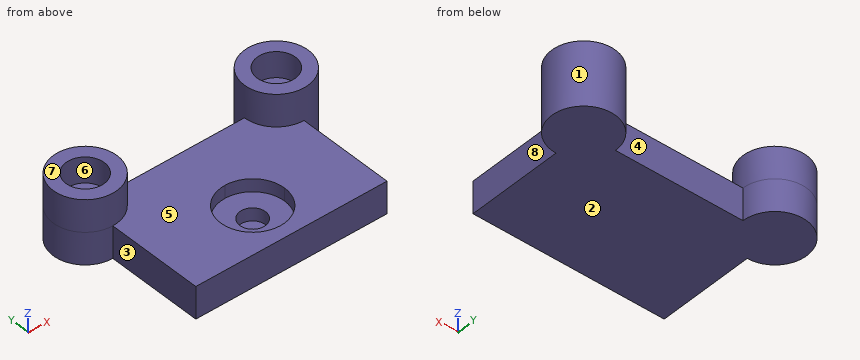
```python
from build123d import *

# Parameters (mm, degrees)
SKETCH_1_W          = 150
SKETCH_1_H          = 100
EXTRUDE_1_DEPTH     = 25
SKETCH_2_R          = 25
EXTRUDE_2_DEPTH     = 25
SKETCH_3_R          = 15
CUT_EXTRUDE_1_DEPTH = 20
SKETCH_4_R          = 7.5
CUT_EXTRUDE_2_DEPTH = 15
CUT_EXTRUDE_3_DEPTH = 10
SKETCH_6_R          = 10
CUT_EXTRUDE_4_DEPTH = 10


with BuildPart() as part:
    # Эскиз1 → Бобышка-Вытянуть1 (new body)
    with BuildSketch(Plane.XY):
        with Locations((75, -50)):
            Rectangle(SKETCH_1_W, SKETCH_1_H)
    extrude(amount=EXTRUDE_1_DEPTH)

    # Эскиз2 → Бобышка-Вытянуть2 (add, symmetric)
    with BuildSketch(Plane.XY.offset(25)):
        Circle(SKETCH_2_R)
        with Locations(Location((150, 0, 0), (0, 0, 180))):
            Circle(SKETCH_2_R)
    extrude(amount=EXTRUDE_2_DEPTH, both=True)

    # Эскиз3 → Вырез-Вытянуть1 (cut)
    with BuildSketch(Plane.XY.offset(50)):
        Circle(SKETCH_3_R)
        with Locations(Location((150, 0, 0), (0, 0, 180))):
            Circle(SKETCH_3_R)
    extrude(amount=-CUT_EXTRUDE_1_DEPTH, mode=Mode.SUBTRACT)

    # Эскиз4 → Вырез-Вытянуть2 (cut)
    with BuildSketch(Plane.XY.offset(30)):
        Circle(SKETCH_4_R)
        with Locations(Location((150, 0, 0), (0, 0, 180))):
            Circle(SKETCH_4_R)
    extrude(amount=-CUT_EXTRUDE_2_DEPTH, mode=Mode.SUBTRACT)

    # Эскиз5 → Вырез-Вытянуть3 (cut)
    with BuildSketch(Plane.XY.offset(25)):
        with BuildLine():
            ThreePointArc((100, -65), (92.67766953, -47.32233047), (75, -40))
            Line((75, -40), (75, -90))
            ThreePointArc((75, -90), (92.67766953, -82.67766953), (100, -65))
        make_face()
        with BuildLine():
            Line((75, -90), (75, -40))
            ThreePointArc((75, -40), (50, -65), (75, -90))
        make_face()
    extrude(amount=-CUT_EXTRUDE_3_DEPTH, mode=Mode.SUBTRACT)

    # Эскиз6 → Вырез-Вытянуть4 (cut)
    with BuildSketch(Plane.XY.offset(15)):
        with Locations((75, -65)):
            Circle(SKETCH_6_R)
    extrude(amount=-CUT_EXTRUDE_4_DEPTH, mode=Mode.SUBTRACT)


solid = part.part
```
Part model, mm, in its own coordinate system. Face numbers are marked on the shaded views. A direction names the side the tool comes from. Round coordinates to 2 decimals unless told otherwise and drop trailing zeros. Loops run counter-clockwise (first coordinate to the right, second up) from the corner with the lowest first, then second, coordinate; pieces in that order, holes last. Notation, with made-up numbers: (-11, 39) -> (-3, 39) arc R22 ccw to (-3, 63) -> close; hole circle Ø4 at (-37.75, 25). An arc over 180 degrees is marked (long way). Use a Markdown table: item, result.
1) Cut at B-B, the plane y = 12. List the corners of the cut face in (x, z).
The answers:
| item | result |
|---|---|
| outline | (-21.93, 0) -> (21.93, 0) -> (21.93, 50) -> (9, 50) -> (9, 30) -> (-9, 30) -> (-9, 50) -> (-21.93, 50) -> close; (128.07, 0) -> (171.93, 0) -> (171.93, 50) -> (159, 50) -> (159, 30) -> (141, 30) -> (141, 50) -> (128.07, 50) -> close |
2) Pull direction X, two halves, no side cores. Call the marked faces 5, 6, 7 and 8: pulls with the +X half, pulls with the -X half, needs draft (parallel to the pull), parting line crosses it, or undercut.
The answers:
| item | result |
|---|---|
| face 5 | undercut |
| face 6 | undercut |
| face 7 | needs draft |
| face 8 | pulls with the +X half |
3) Tool access for the marked faces 1, 2, 3 and 4: list every direction of +Z, -Z, +X, -X, +Y, -Y with a clear straight run to the whole face (end or side of a thin tool).
The answers:
| item | result |
|---|---|
| face 1 | +Z |
| face 2 | -Z, +X, -X, +Y, -Y |
| face 3 | +Z, -Z, -X, -Y |
| face 4 | +Z, -Z, +Y |
4) Drop flat-ended pins along their axis: pin 1 Ø7.5 at (y, z) = (-61, 7) entering from -X; pin 2 Ø15 at (x, y) = (79.5, -53) entering from +Z; pin 3 Ø16.5 at (x, y) = (152, -0.5) entering from +Z. Give the stop position or say it passes through.
The answers:
| item | result |
|---|---|
| pin 1 | stops at x = 0 |
| pin 2 | stops at z = 15 |
| pin 3 | stops at z = 30 |
5) Cut at D-D, the plane x = -3. List the corners of the cut face in (y, z).
The answers:
| item | result |
|---|---|
| outline | (-24.82, 0) -> (24.82, 0) -> (24.82, 50) -> (14.7, 50) -> (14.7, 30) -> (6.87, 30) -> (6.87, 15) -> (-6.87, 15) -> (-6.87, 30) -> (-14.7, 30) -> (-14.7, 50) -> (-24.82, 50) -> close |
6) Probe line 1 (Y direction, x = 75, z = 10.25); line 2 (Y direction, x = 150, z = 36); line 3 (Z direction, x = 97, y = -81). List the from-to ranges inside material, lowest first. Write a range as [from, to].
The answers:
| item | result |
|---|---|
| line 1 | y = [-100, -75], [-55, 0] |
| line 2 | y = [-25, -15], [15, 25] |
| line 3 | z = [0, 25] |
7) Cut at A-A, the plane z = 43.5. List the corners of the cut face in (x, y), and give its area (3 significant figures).
The answers:
| item | result |
|---|---|
| outline | circle Ø50 at (0, 0); circle Ø50 at (150, 0); hole circle Ø30 at (0, 0); hole circle Ø30 at (150, 0) |
| area | 2,510 mm2 |
8) Cut at C-C, the plane y = -71.5. List the corners of the cut face in (x, z).
The answers:
| item | result |
|---|---|
| outline | (0, 0) -> (150, 0) -> (150, 25) -> (99.14, 25) -> (99.14, 15) -> (82.6, 15) -> (82.6, 5) -> (67.4, 5) -> (67.4, 15) -> (50.86, 15) -> (50.86, 25) -> (0, 25) -> close |
